from build123d import *

# Parameters (mm, degrees)
BOSS_EXTRUDE1_DEPTH = 5
SKETCH2_R           = 1.7
CUT_EXTRUDE1_DEPTH  = 19.809904306
SKETCH3_R           = 1.7
CUT_EXTRUDE2_DEPTH  = 14.849638984


with BuildPart() as part:
    # Sketch1 → Boss-Extrude1 (new body)
    with BuildSketch(Plane(origin=(0, 0, 0), x_dir=(0, 0, -1), z_dir=(1, 0, 0))):
        Polygon((-4.75, -7.25), (-4.75, -8.75), (4.75, -8.75), (4.75, 8.75), (3.25, 8.75), (3.25, -7.25), align=None)
    extrude(amount=BOSS_EXTRUDE1_DEPTH)

    # Sketch2 → Cut-Extrude1 (cut, through all)
    with BuildSketch(Plane.XZ.offset(8.75)):
        with Locations(Location((2.5, 2.25, 0), (0, 0, 270))):
            Circle(SKETCH2_R)
    extrude(amount=-CUT_EXTRUDE1_DEPTH, mode=Mode.SUBTRACT)

    # Sketch3 → Cut-Extrude2 (cut, through all)
    with BuildSketch(Plane(origin=(0, 0, -4.75), x_dir=(-1, 0, 0), z_dir=(0, 0, -1))):
        with Locations((-2.5, -1.75)):
            Circle(SKETCH3_R)
        with Locations((-2.5, 6.25)):
            Circle(SKETCH3_R)
    extrude(amount=-CUT_EXTRUDE2_DEPTH, mode=Mode.SUBTRACT)


solid = part.part
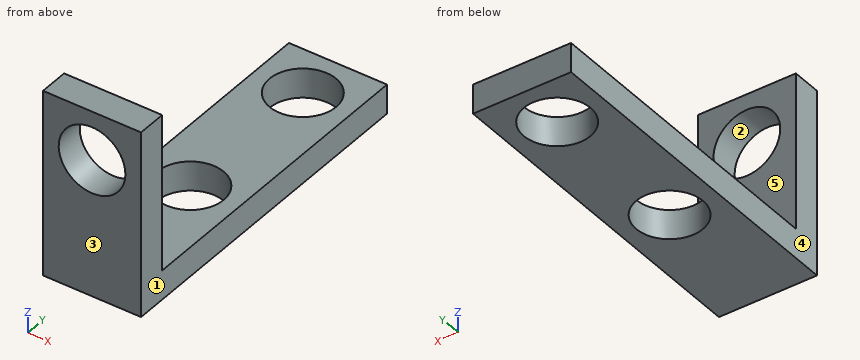
Part model, mm, in its own coordinate system. Face numbers are marked on the shaded views. A direction names the side the tool comes from. Round coordinates to 2 decimals unless told otherwise and drop trailing zeros. Write each loop counter-clockwise with the first axis right and the second up, starting at its lowest first coordinate (ties: lowest second). Pieces come first, ordered by that corner, then holes. Notation, with made-up numbers: (71.5, 42) - (115.5, 42) arc R35 ccw to (115.5, 78) - close; hole circle Ø8 at (78, 49). An arc over 180 degrees is marked (long way). Use CSV: the item, a comma, the result in double quotes.
Item 1: Wall check: L1, parallel to Y at x = 2.5, z = -3.8; L2, parallel to X at y = -7.65, z = 2.25; L3, parallel to Y at x = 0.4, z = 2.25. Give the ranges that are in metal, low to high.
Results list:
L1,"y = -8.75 to -3.45, -0.05 to 4.55, 7.95 to 8.75"
L2,"x = 0 to 0.8, 4.2 to 5"
L3,"y = -8.75 to -7.25"
Item 2: Slice it at D-D, the plane x = 3.3. Write the cut outline in (y, z).
Results list:
outline,"(-8.75, -4.75) - (-3.25, -4.75) - (-3.25, -3.25) - (-7.25, -3.25) - (-7.25, 0.75) - (-8.75, 0.75) - close; (-8.75, 3.75) - (-7.25, 3.75) - (-7.25, 4.75) - (-8.75, 4.75) - close; (-0.25, -4.75) - (4.75, -4.75) - (4.75, -3.25) - (-0.25, -3.25) - close; (7.75, -4.75) - (8.75, -4.75) - (8.75, -3.25) - (7.75, -3.25) - close"
Item 3: Slice it at C-C, the plane z = 2.25. Write the cut outline in (x, y), then the cut area to 3 significant figures.
Results list:
outline,"(0, -8.75) - (0.8, -8.75) - (0.8, -7.25) - (0, -7.25) - close; (4.2, -8.75) - (5, -8.75) - (5, -7.25) - (4.2, -7.25) - close"
area,"2.40 mm²"
Item 4: Flat gauge pins, fed straight in: P1, Ø2, axis at x = 1, y = -3.5, coming from the +Z side; P2, Ø2, axis at x = 2.5, y = -1.75, coming from the -Z side. Where does each tip first touch, or does it go through?
Results list:
P1,"stops at z = -3.25"
P2,"passes through"
Item 5: Tool access for the marked faces 4 and 5: list every direction of +Z, -Z, +X, -X, +Y, -Y with a clear straight run to the whole face (end or side of a thin tool).
Results list:
face 4,"+Z, -Z, -X, +Y, -Y"
face 5,"+Z, +X, -X, +Y"
Item 6: Slice it at B-B, the plane y = 6.25. Write the cut outline in (x, z).
Results list:
outline,"(0, -4.75) - (0.8, -4.75) - (0.8, -3.25) - (0, -3.25) - close; (4.2, -4.75) - (5, -4.75) - (5, -3.25) - (4.2, -3.25) - close"
Item 7: Pull direction X, two halves, no side cores. Call the marked faces 1, 2 and 3: pulls with the +X half, pulls with the -X half, needs draft (parallel to the pull), parting line crosses it, or undercut.
Results list:
face 1,"pulls with the +X half"
face 2,"undercut"
face 3,"needs draft"
Item 8: Slice it at A-A, the plane x = 2.5. Write the cut outline in (y, z).
Results list:
outline,"(-8.75, -4.75) - (-3.45, -4.75) - (-3.45, -3.25) - (-7.25, -3.25) - (-7.25, 0.55) - (-8.75, 0.55) - close; (-8.75, 3.95) - (-7.25, 3.95) - (-7.25, 4.75) - (-8.75, 4.75) - close; (-0.05, -4.75) - (4.55, -4.75) - (4.55, -3.25) - (-0.05, -3.25) - close; (7.95, -4.75) - (8.75, -4.75) - (8.75, -3.25) - (7.95, -3.25) - close"
